Input: part model. Units: mm. Frame: model coordinates. Face numbers are marked on the shaded views. A direction names the side the tool comes from. Coordinates: 2 decimals unless noted, no trailing zeros. Write each loop counter-clockwise with the first axis right and the second up, starting at its lowest first coordinate (ties: lowest second). Pieces come first, ordered by that corner, then holes. Notation, with made-up numbers: (-0.75, 24) - (7.25, 24) arc R19 cw to (7.25, 31) - close; hole circle Ø1 at (51.25, 73). An arc over 180 degrees is marked (long way). One line per question, with ' | ' between items. Start each with the question number.
1) Section query A-A on x = 56.5. Return loops of the section in (y, z), and give its area (3 significant figures).
2) Section query D-D on z = 30. Return loops of the section in (x, y).
3) Draft query along Y for the marked faces 1, 2 and 3. Return one class per face: released by +Y, released by -Y, zero draft, split by the parting line, or undercut.
4) First-contact query: P1, Ø6.5, axis at y = 16.5, z = 52, coming from the -X side; P2, Ø6, axis at x = -34, y = 56, coming from the -Z side; P3, Ø6.5, axis at y = 92, z = 49.5, coming from the -X side. Flat tips, straight axial feed; report the tip coordinate or a pass-through.
5) Reachability of the marked faces 4 and 5 from +Z, -Z, +X, -X, +Y, -Y: full face, straight path, thin tool, end or side. Return the list, or none.
6) Section query B-B on y = 14.5. Return loops of the section in (x, z), and give its area (3 significant figures).
7) Line query: line 1 (X direction, y = 50, z = 44); line 2 (X direction, y = 50, z = 45); line 3 (Z direction, x = 95.5, y = 41.5). Output: solid intervals per line, ascending.
8) Section query C-C on y = 50. Return loops of the section in (x, z).
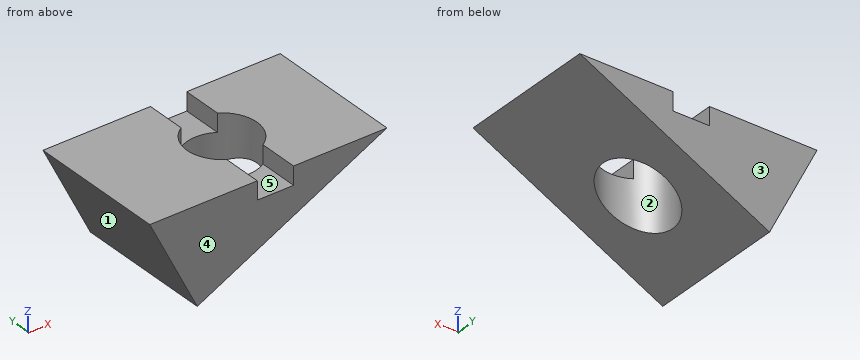
```python
from build123d import *

# Parameters (mm, degrees)
ESTRUSIONE_ESTRUSIONE1_DEPTH = 100
TAGLIO_ESTRUSIONE2_DEPTH     = 13
SCHIZZO5_R                   = 25
TAGLIO_ESTRUSIONE3_DEPTH     = 169.564420887


with BuildPart() as part:
    # Schizzo1 → Estrusione-Estrusione1 (new body)
    with BuildSketch(Plane(origin=(0, 0, 0), x_dir=(1, 0, 0), z_dir=(0, 1, 0))):
        Polygon((-52.496864645, -55.39158852), (117.444301645, -55.39158852), (-18.508631387, 12.584877996), align=None)
    extrude(amount=ESTRUSIONE_ESTRUSIONE1_DEPTH)

    # Schizzo2 → Taglio-Estrusione2 (cut)
    with BuildSketch(Plane.XY.offset(55.39158852)):
        with BuildLine():
            Line((50.503135355, 100), (37.503135355, 100))
            Line((37.503135355, 100), (37.503135355, 75))
            ThreePointArc((37.503135355, 75), (44.253916325, 74.071289045), (50.503135355, 71.354156504))
            Line((50.503135355, 71.354156504), (50.503135355, 100))
        make_face()
        with BuildLine():
            Line((37.503135355, 75), (37.503135355, 100))
            Line((37.503135355, 100), (24.503135355, 100))
            Line((24.503135355, 100), (24.503135355, 71.354156504))
            ThreePointArc((24.503135355, 71.354156504), (30.752354386, 74.071289045), (37.503135355, 75))
        make_face()
        with BuildLine():
            ThreePointArc((50.503135355, 28.645843496), (44.253916325, 25.928710955), (37.503135355, 25))
            Line((37.503135355, 25), (37.503135355, 0))
            Line((37.503135355, 0), (50.503135355, 0))
            Line((50.503135355, 0), (50.503135355, 28.645843496))
        make_face()
        with BuildLine():
            Line((37.503135355, 0), (37.503135355, 25))
            ThreePointArc((37.503135355, 25), (30.752354386, 25.928710955), (24.503135355, 28.645843496))
            Line((24.503135355, 28.645843496), (24.503135355, 0))
            Line((24.503135355, 0), (37.503135355, 0))
        make_face()
    extrude(amount=-TAGLIO_ESTRUSIONE2_DEPTH, mode=Mode.SUBTRACT)

    # Schizzo5 → Taglio-Estrusione3 (cut, through all)
    with BuildSketch(Plane.XY.offset(55.39158852)):
        with Locations((37.503135355, 50)):
            Circle(SCHIZZO5_R)
    extrude(amount=-TAGLIO_ESTRUSIONE3_DEPTH, mode=Mode.SUBTRACT)


solid = part.part
```
Answer key:
1) outline: (0, 24.92) - (33.75, 24.92) - (33.75, 55.39) - (0, 55.39) - close; (66.25, 24.92) - (100, 24.92) - (100, 55.39) - (66.25, 55.39) - close | area: 2,060 mm²
2) outline: (-39.8, 0) - (66.66, 0) - (66.66, 100) - (-39.8, 100) - close; hole circle Ø50 at (37.5, 50)
3) face 1: zero draft | face 2: undercut | face 3: released by +Y
4) P1: x = -52.43 | P2: z = 12.4 | P3: x = -51.18
5) face 4: +Z, -Z, +X, -X, -Y | face 5: +Z, +Y, -Y
6) outline: (-52.5, 55.39) - (-18.51, -12.58) - (117.44, 55.39) - (50.5, 55.39) - (50.5, 42.39) - (24.5, 42.39) - (24.5, 55.39) - close | area: 5,440 mm²
7) line 1: -46.8 to 12.5, 62.5 to 94.66 | line 2: -47.3 to 12.5, 62.5 to 96.66 | line 3: 44.42 to 55.39
8) outline: (-52.5, 55.39) - (-18.51, -12.58) - (12.5, 2.92) - (12.5, 55.39) - close; (62.5, 27.92) - (117.44, 55.39) - (62.5, 55.39) - close
